Read the model definition and answer for the solid it produces. Units are mm, in the model's axes. A direction names the side the tool comes from. Round coordinates to 2 decimals unless told otherwise and drop trailing zeros. Order: outer loops, then holes, each group sorted by start corner. A loop starts at its lowest first (then second) coordinate and runs counter-clockwise, first axis right, second up. Notation, with made-up numbers: (-4, 25.25) -> (4, 25.25) arc R29 ccw to (4, 56.25) -> close; hole circle Ø2 at (-30, 65.5). An arc over 180 degrees is marked (long way). Use a Markdown table: item, result. Add a question column.
1. Consider L1, parallel to X at y = 5.75, z = -60; L2, parallel to Y at x = 44.5, z = 22.5; L3, parallel to X at y = 19, z = -1. Determine where each line is inside the solid, lowest interval first. Write a range as [from, to].
2. Section D-D, the plane x = 55 is taken. Give the vertices of the cut face in (y, z), then the cut area to 3 significant figures.
3. Section B-B, the plane z = -2 is taken. Give the vertices of the cut face in (x, y).
4. Given pin 1 (4 mm diameter, centred on x = 6, y = 25, fed in from -Z); pin 2 (5 mm diameter, centred on x = -0.5, y = 17, fed in from -Z); pin 3 (5.5 mm diameter, centred on x = -60, z = -60, fed in from +Y), each flat-ended and moving along its own axis, determine where each tip first touches the part or whether it passes through.
5. For faces 4 (the face through (-4.88, 19.86, -1.08)), 5 (the face through (-59.93, 4.93, -61.7)), determine the directions among +Z, -Z, +X, -X, +Y, -Y from which every point of the face is accessible in a straight line to the end or side of a thin tool.
6. Section C-C, the plane y = 19.5 is taken. Give the vertices of the cut face in (x, z), then the cut area to 3 significant figures.
7. The mould has two halves that part along Z. Classify faces 1 (the face through (60.07, 4.93, -61.7)), 2 (the face through (-1, 5, -75)), 3 (the face through (75, 5, 1)): +Z half, -Z half, draft (parallel to the pull), parting line (faces both ways), or undercut.
8. Section A-A, the plane x = 0 is taken. Give the vertices of the cut face in (y, z), then the cut area to 3 significant figures.
```python
from build123d import *

# Parameters (mm, degrees)
SKETCH2_W           = 150
SKETCH2_H           = 150
SKETCH2_R           = 1.7
SKETCH2_R_2         = 5
BOSS_EXTRUDE1_DEPTH = 10
SKETCH2_3_R         = 5
BOSS_EXTRUDE2_DEPTH = 30


with BuildPart() as part:
    # Sketch2 → Boss-Extrude1 (new body)
    with BuildSketch(Plane(origin=(0, 0, 0), x_dir=(1, 0, 0), z_dir=(0, 1, 0))):
        Rectangle(SKETCH2_W, SKETCH2_H)
        with Locations(Location((-60, 60, 0), (0, 0, 270))):
            Circle(SKETCH2_R, mode=Mode.SUBTRACT)
        with Locations(Location((60, 60, 0), (0, 0, 270))):
            Circle(SKETCH2_R, mode=Mode.SUBTRACT)
        with Locations(Location((60, -60, 0), (0, 0, 270))):
            Circle(SKETCH2_R, mode=Mode.SUBTRACT)
        with Locations(Location((-60, -60, 0), (0, 0, 270))):
            Circle(SKETCH2_R, mode=Mode.SUBTRACT)
        with Locations(Location((0, 0, 0), (0, 0, 270))):
            Circle(SKETCH2_R_2, mode=Mode.SUBTRACT)
    extrude(amount=BOSS_EXTRUDE1_DEPTH)

    # Sketch2_3 → Boss-Extrude2 (add)
    with BuildSketch(Plane(origin=(0, 0, 0), x_dir=(1, 0, 0), z_dir=(0, 1, 0))):
        with Locations(Location((0, 0, 0), (0, 0, 270))):
            Circle(SKETCH2_3_R)
    extrude(amount=BOSS_EXTRUDE2_DEPTH)


solid = part.part
```
Verdict:
| question | item | result |
|---|---|---|
| 1 | L1 | x = [-75, -61.7], [-58.3, 58.3], [61.7, 75] |
| 1 | L2 | y = [0, 10] |
| 1 | L3 | x = [-4.9, 4.9] |
| 2 | outline | (0, -75) -> (10, -75) -> (10, 75) -> (0, 75) -> close |
| 2 | area | 1,500 mm2 |
| 3 | outline | (-75, 0) -> (75, 0) -> (75, 10) -> (4.58, 10) -> (4.58, 30) -> (-4.58, 30) -> (-4.58, 10) -> (-75, 10) -> close |
| 4 | pin 1 | stops at z = -3 |
| 4 | pin 2 | stops at z = -5 |
| 4 | pin 3 | stops at y = 10 |
| 5 | face 4 | +Y |
| 5 | face 5 | +Y, -Y |
| 6 | outline | circle Ø10 at (0, 0) |
| 6 | area | 78.5 mm2 |
| 7 | face 1 | undercut |
| 7 | face 2 | -Z half |
| 7 | face 3 | draft |
| 8 | outline | (0, -75) -> (10, -75) -> (10, -5) -> (30, -5) -> (30, 5) -> (10, 5) -> (10, 75) -> (0, 75) -> close |
| 8 | area | 1,700 mm2 |
